For this review, take the finished solid that the model builds, in its own axes (mm). A direction names the side the tool comes from. Round coordinates to 2 decimals unless told otherwise and drop trailing zeros. Write each loop counter-clockwise with the first axis right and the second up, starting at its lowest first coordinate (ties: lowest second). Pieces come first, ordered by that corner, then holes. Notation, with made-up numbers: (84, 54.5) -> (117, 54.5) arc R23 cw to (117, 86.5) -> close; hole circle Ø3 at (33, 45.5). An arc over 180 degrees is marked (long way). Answer in a Markdown table with one row per item.
from build123d import *

# Parameters (mm, degrees)
F0_W     = 57.15
F0_H     = 19.05
F1_DEPTH = 19.05
F2_W     = 19.05
F2_H     = 19.05
F3_DEPTH = 19.05
F4_W     = 19.05
F4_H     = 19.05
F5_DEPTH = 19.05
F7_DEPTH = 38.1


with BuildPart() as f1:
    # F0 (on Front) → F1 (new body)
    with BuildSketch(Plane.XZ):
        with Locations((28.575, 9.525)):
            Rectangle(F0_W, F0_H)
    extrude(amount=F1_DEPTH)

    # F4 (on face) → F5 (join)
    with BuildSketch(Plane.XZ.offset(19.05)):
        with Locations((9.525, 9.525)):
            Rectangle(F4_W, F4_H)
    extrude(amount=F5_DEPTH)



with BuildPart() as f3:
    # F2 (on face) → F3 (new body)
    with BuildSketch(Plane.XZ.offset(19.05)):
        with Locations((47.625, 9.525)):
            Rectangle(F2_W, F2_H)
    extrude(amount=F3_DEPTH)


with BuildPart() as f1_1:
    add(f1.part)

    add(f3.part)  # F7 merges F3
    # F6 (on Top) + F5_face (on face) → F7 (join)
    with BuildSketch(Plane.XY):
        Polygon((0, -19.164518), (0, -38.021836), (19.069996, -38.098183), (19.069996, -19.164518), align=None)
    with BuildSketch(Plane(origin=(23.8125, -14.2875, 19.05), x_dir=(1, 0, 0), z_dir=(0, 0, 1))):
        Polygon((33.3375, -4.7625), (33.3375, 14.2875), (-23.8125, 14.2875), (-23.8125, -23.8125), (-4.7625, -23.8125), (-4.7625, -4.7625), align=None)
    extrude(amount=F7_DEPTH)


solid = f1_1.part
1) Mouldability with a two-part tool opening along X and no side actions: class faces 4 (the flat face through (0, -19, 28)), 5 (the flat face through (47, -38.1, 10)), 6 (the flat face through (19.07, -29, 19)) as pulls with the +X half, pulls with the -X half, needs draft (parallel to the pull), parting line crosses it, or undercut.
Solved:
| item | result |
|---|---|
| face 4 | pulls with the -X half |
| face 5 | needs draft |
| face 6 | undercut |
2) For faces 1 (the flat face through (57.15, -15, 22)), 2 (the flat face through (47, -28, 19.05)), 3 (the flat face through (38.1, -28, 9)), list the 3-axis set-ups (+Z, -Z, +X, -X, +Y, -Y) from which the entire face can be reached by the end or side of a thin tool; tool diameter is ignored.
Solved:
| item | result |
|---|---|
| face 1 | +Z, -Z, +X, +Y, -Y |
| face 2 | +Z, +X, -Y |
| face 3 | +Z, -Z, -Y |
3) Clearance check with a flat-ended pin moving along its axis: pin 1 Ø5.5 at (x, y) = (43, -24) entering from +Z. State where the tip first meets the part, or that it passes through.
Solved:
| item | result |
|---|---|
| pin 1 | z = 19.05 |
4) Consider section C-C on x = 47. State the section outline as (y, z) points, then the cut area to 3 significant figures.
Solved:
| item | result |
|---|---|
| outline | (-38.1, 0) -> (0, 0) -> (0, 57.15) -> (-19.05, 57.15) -> (-19.05, 19.05) -> (-38.1, 19.05) -> close |
| area | 1,450 mm² |
5) For line 1 (X direction, y = -25.5, z = 15); line 2 (Z direction, x = 55.5, y = -32.5); line 3 (Y direction, x = 52, z = 35.5), list the stretches that pass through material, from the lowest coordinate up. Write a range as [from, to].
Solved:
| item | result |
|---|---|
| line 1 | [0, 19.07], [38.1, 57.15] |
| line 2 | [0, 19.05] |
| line 3 | [-19.05, 0] |
